```python
from build123d import *

# Parameters (mm, degrees)
SKETCH1_W           = 60
SKETCH1_H           = 60
BOSS_EXTRUDE1_DEPTH = 60
SKETCH3_W           = 30
SKETCH3_H           = 20
CUT_EXTRUDE1_DEPTH  = 20
SKETCH4_W           = 30
SKETCH4_H           = 20
CUT_EXTRUDE2_DEPTH  = 20
BOSS_EXTRUDE2_DEPTH = 30
CUT_EXTRUDE3_DEPTH  = 30
CUT_EXTRUDE4_DEPTH  = 30
CUT_EXTRUDE6_DEPTH  = 0.0001
CUT_EXTRUDE7_DEPTH  = 0.0001


with BuildPart() as part:
    # Sketch1 → Boss-Extrude1 (new body)
    with BuildSketch(Plane.XY):
        with Locations((30, 30)):
            Rectangle(SKETCH1_W, SKETCH1_H)
    extrude(amount=BOSS_EXTRUDE1_DEPTH)

    # Sketch3 → Cut-Extrude1 (cut)
    with BuildSketch(Plane(origin=(0, 60, 0), x_dir=(1, 0, 0), z_dir=(0, 1, 0))):
        with Locations((15, -10)):
            Rectangle(SKETCH3_W, SKETCH3_H)
    extrude(amount=-CUT_EXTRUDE1_DEPTH, mode=Mode.SUBTRACT)

    # Sketch4 → Cut-Extrude2 (cut)
    with BuildSketch(Plane(origin=(0, 60, 0), x_dir=(1, 0, 0), z_dir=(0, 1, 0))):
        with Locations((15, -50)):
            Rectangle(SKETCH4_W, SKETCH4_H)
    extrude(amount=-CUT_EXTRUDE2_DEPTH, mode=Mode.SUBTRACT)

    # Sketch5 → Boss-Extrude2 (add)
    with BuildSketch(Plane.ZY):
        Polygon((60, 40), (40, 60), (40, 40), align=None)
        Polygon((0, 40), (20, 40), (20, 60), align=None)
    extrude(amount=-BOSS_EXTRUDE2_DEPTH)

    # Sketch6 → Cut-Extrude3 (cut)
    with BuildSketch(Plane.ZY):
        Polygon((60, 20), (40, 0), (60, 0), align=None)
    extrude(amount=-CUT_EXTRUDE3_DEPTH, mode=Mode.SUBTRACT)

    # Sketch7 → Cut-Extrude4 (cut)
    with BuildSketch(Plane.ZY):
        Polygon((0, 20), (20, 0), (0, 0), align=None)
    extrude(amount=-CUT_EXTRUDE4_DEPTH, mode=Mode.SUBTRACT)

    # Sketch8 → Cut-Extrude6 (cut)
    with BuildSketch(Plane(origin=(0, 60, 0), x_dir=(1, 0, 0), z_dir=(0, 1, 0))):
        with BuildLine():
            Line((30, -60), (30, 0))
            ThreePointArc((30, 0), (60, -30), (30, -60))
        make_face()
    extrude(amount=-CUT_EXTRUDE6_DEPTH, mode=Mode.SUBTRACT)

    # Sketch9 → Cut-Extrude7 (cut)
    with BuildSketch(Plane.XY.offset(60)):
        with BuildLine():
            Line((30, 0), (30, 60))
            ThreePointArc((30, 60), (60, 30), (30, 0))
        make_face()
    extrude(amount=-CUT_EXTRUDE7_DEPTH, mode=Mode.SUBTRACT)


solid = part.part
```
Design review of the part built by this model. Coordinates are the model's own, in mm. A direction names the side the tool comes from. Coordinates: 2 decimals unless noted, no trailing zeros. Loops run counter-clockwise (first coordinate to the right, second up) from the corner with the lowest first, then second, coordinate; pieces in that order, holes last. Notation, with made-up numbers: (61, 50.25) -> (120, 50.25) arc R27 cw to (120, 69.25) -> close; hole circle Ø9 at (35, -15.75). An arc over 180 degrees is marked (long way). Answer as a JSON object with one key per item and string values.
Q1. Take a section at C-C on x = 14.5. Give the boundary of the cut face in (y, z), plus the area to 3 significant figures.
Answer block:
{"outline": "(0, 20) -> (20, 0) -> (40, 0) -> (60, 20) -> (60, 40) -> (40, 60) -> (20, 60) -> (0, 40) -> close", "area": "2,800 mm^2"}
Q2. Clearance check with flat-ended pins moving along their axes: pin 1 Ø1 at (x, y) = (7.5, 41.5) entering from +Z; pin 2 Ø10 at (x, z) = (10, 12) entering from +Y; pin 3 Ø10 at (y, z) = (53.5, 5.5) entering from -X. State where each tip first meets the part, or that it passes through.
Answer block:
{"pin 1": "stops at z = 59", "pin 2": "stops at y = 57", "pin 3": "stops at x = 30"}
Q3. To check wall thickness, follow L1, parallel to X at y = 12.5, z = 7; L2, parallel to Y at x = 29.5, z = 43; L3, parallel to Y at x = 24.5, z = 4.5. State the ranges of each line that lie inside material, in increasing order.
Answer block:
{"L1": "x = 30 to 60", "L2": "y = 3 to 57", "L3": "y = 15.5 to 44.5"}
Q4. Tool access review of faces 1 (the flat face through (15, 50, 50)), 2 (the flat face through (30, 55, 6)), 3 (the flat face through (15, 10, 50)): name each direction out of +Z, -Z, +X, -X, +Y, -Y from which nothing blocks a thin tool from reaching the whole face with its end or side.
Answer block:
{"face 1": "+Z, -X, +Y", "face 2": "-Z, -X, +Y", "face 3": "+Z, -X, -Y"}
